Check sheet for the modelled part. Datum: model origin and axes. Units: mm. Face numbers are marked on the shaded views. A direction names the side the tool comes from. Give positions to 0.01 mm unless a question says otherwise; leave off trailing zeros. Loops run counter-clockwise (first coordinate to the right, second up) from the corner with the lowest first, then second, coordinate; pieces in that order, holes last. Notation, with made-up numbers: (-10, 68) - (37, 68) arc R24 cw to (37, 85) - close; hole circle Ø5 at (-39.75, -35.75). An arc over 180 degrees is marked (long way). Use CSV: the item, a comma, the result in double quotes.
from build123d import *

# Parameters (mm, degrees)
F0_R     = 2.3876
F1_DEPTH = 3.81
F2_R     = 2.3876
F3_DEPTH = 3.81
F4_SIZE  = 1.27


with BuildPart() as f1:
    # F0 (on Top) → F1 (new body)
    with BuildSketch(Plane.XY):
        with BuildLine():
            ThreePointArc((5.715, 9.7989101959), (0, 7.9772757461), (-5.715, 9.7989101959))
            Line((-5.715, 9.7989101959), (-5.715, 19.3437465092))
            Line((-5.715, 19.3437465092), (-7.6151215981, 19.3437465092))
            Line((-7.6151215981, 19.3437465092), (-9.3965170219, 13.432749836))
            Line((-9.3965170219, 13.432749836), (-9.3965170219, 6.983557897))
            Line((-9.3965170219, 6.983557897), (-4.1960714835, 1.5722833676))
            Line((-4.1960714835, 1.5722833676), (-4.1960714835, -12.9142534908))
            ThreePointArc((-4.1960714835, -12.9142534908), (-3.0057534422, -15.7879354495), (-0.1320714835, -16.9782534908))
            Line((-0.1320714835, -16.9782534908), (0, -16.9782534908))
            Line((0, -16.9782534908), (0.1320714835, -16.9782534908))
            ThreePointArc((0.1320714835, -16.9782534908), (3.0057534422, -15.7879354495), (4.1960714835, -12.9142534908))
            Line((4.1960714835, -12.9142534908), (4.1960714835, 1.5722833676))
            Line((4.1960714835, 1.5722833676), (9.3965170219, 6.983557897))
            Line((9.3965170219, 6.983557897), (9.3965170219, 13.432749836))
            Line((9.3965170219, 13.432749836), (7.6151215981, 19.3437465092))
            Line((7.6151215981, 19.3437465092), (5.715, 19.3437465092))
            Line((5.715, 19.3437465092), (5.715, 9.7989101959))
        make_face()
        with Locations((0, -11.8050774974)):
            Circle(F0_R, mode=Mode.SUBTRACT)
    extrude(amount=F1_DEPTH)

    # F2 (on face) → F3 (join)
    with BuildSketch(Plane.XY.offset(3.81)):
        with BuildLine():
            Line((-5.715, 9.7989101959), (-5.715, 19.3437465092))
            Line((-5.715, 19.3437465092), (-7.6151215981, 19.3437465092))
            Line((-7.6151215981, 19.3437465092), (-9.3965170219, 13.432749836))
            Line((-9.3965170219, 13.432749836), (-9.3965170219, 6.983557897))
            Line((-9.3965170219, 6.983557897), (-4.1960714835, 1.5722833676))
            Line((-4.1960714835, 1.5722833676), (-4.1960714835, -12.9142534908))
            ThreePointArc((-4.1960714835, -12.9142534908), (-3.0057534422, -15.7879354495), (-0.1320714835, -16.9782534908))
            Line((-0.1320714835, -16.9782534908), (0.1320714835, -16.9782534908))
            ThreePointArc((0.1320714835, -16.9782534908), (3.0057534422, -15.7879354495), (4.1960714835, -12.9142534908))
            Line((4.1960714835, -12.9142534908), (4.1960714835, 1.5722833676))
            Line((4.1960714835, 1.5722833676), (9.3965170219, 6.983557897))
            Line((9.3965170219, 6.983557897), (9.3965170219, 13.432749836))
            Line((9.3965170219, 13.432749836), (7.6151215981, 19.3437465092))
            Line((7.6151215981, 19.3437465092), (5.715, 19.3437465092))
            Line((5.715, 19.3437465092), (5.715, 9.7989101959))
            ThreePointArc((5.715, 9.7989101959), (0, 7.9772757461), (-5.715, 9.7989101959))
        make_face()
        with Locations((0, -11.8050774974)):
            Circle(F2_R, mode=Mode.SUBTRACT)
        with BuildLine():
            Line((-2.9692309909, 19.3437465092), (-5.715, 19.3437465092))
            Line((-5.715, 19.3437465092), (-5.715, 9.7989101959))
            ThreePointArc((-5.715, 9.7989101959), (0, 7.9772757461), (5.715, 9.7989101959))
            Line((5.715, 9.7989101959), (5.715, 19.3437465092))
            Line((5.715, 19.3437465092), (2.9692309909, 19.3437465092))
            Line((2.9692309909, 19.3437465092), (2.9692309909, 10.7184536755))
            Line((2.9692309909, 10.7184536755), (0, 10.7184536755))
            Line((0, 10.7184536755), (-2.9692309909, 10.7184536755))
            Line((-2.9692309909, 10.7184536755), (-2.9692309909, 19.3437465092))
        make_face()
    extrude(amount=F3_DEPTH)

    # F4
    f4_edges = [f1.edges().sort_by_distance(p)[0] for p in [
        (-8.505819, 16.388248, 7.62),
        (-9.396517, 10.208154, 7.62),
        (-6.796294, 4.277921, 7.62),
        (-4.196071, -5.670985, 7.62),
        (6.796294, 4.277921, 7.62),
        (9.396517, 10.208154, 7.62),
        (8.505819, 16.388248, 7.62),
    ]]
    chamfer(f4_edges, length=F4_SIZE)


solid = f1.part
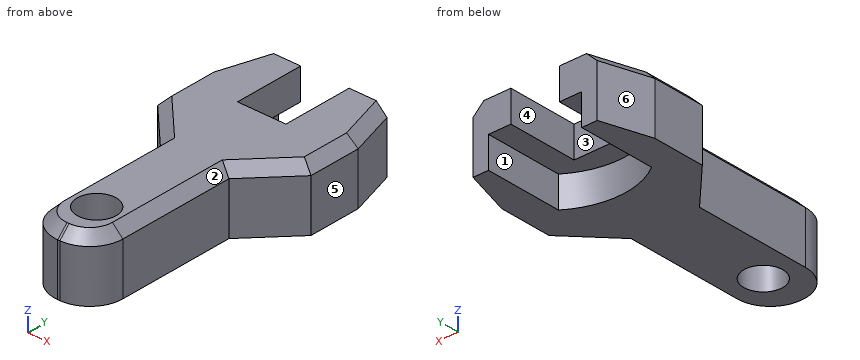
1. Scan lines: line 1 along Y through (x, z) = (0, 5.5); line 2 along X through (y, z) = (-12, 5); line 3 along Z through (x, y) = (-5.25, 12.5). Record each from-to range of solid material in increasing order.
Completed:
line 1,"y = -16.98 to -14.19, -9.42 to 10.72"
line 2,"x = -4.2 to -2.38, 2.38 to 4.2"
line 3,"z = 3.81 to 7.62"
2. Sectioned sample at A-A, the plane y = 15. Record the boundary of the cut face in (x, z) (3 decimals), and give its area (3 significant figures).
Completed:
outline,"(-8.924, 0) - (-5.715, 0) - (-5.715, 3.81) - (-2.969, 3.81) - (-2.969, 7.62) - (-7.598, 7.62) - (-8.924, 6.35) - close; (2.969, 3.81) - (5.715, 3.81) - (5.715, 0) - (8.924, 0) - (8.924, 6.35) - (7.598, 7.62) - (2.969, 7.62) - close"
area,"68.1 mm²"
3. Go/stop test with flat-tipped pins: pin 1 Ø5.5 at (x, y) = (0.5, 12) entering from -Z; pin 2 Ø1.1 at (y, z) = (16, 5) entering from +X; pin 3 Ø3 at (y, z) = (15, 1.5) entering from -X. Record where each tip stops, or that it passes through.
Completed:
pin 1,"stops at z = 3.81"
pin 2,"stops at x = 8.79"
pin 3,"stops at x = -9.38"
4. Sectioned sample at B-B, the plane y = -6. Record the boundary of the cut face in (x, z), and give its area (3 significant figures).
Completed:
outline,"(-4.2, 0) - (4.2, 0) - (4.2, 6.35) - (2.93, 7.62) - (-2.93, 7.62) - (-4.2, 6.35) - close"
area,"62.3 mm²"
5. Release check for a two-part mould opening along X. For the marked faces 4, 5 and 6 record: released by +X, released by -X, zero draft, split by the parting line, or undercut.
Completed:
face 4,"undercut"
face 5,"released by +X"
face 6,"released by -X"
6. Set-up check for the marked faces 1, 2 and 3: record each of +Z, -Z, +X, -X, +Y, -Y from which the full face is reachable in a straight line by a thin tool's end or side.
Completed:
face 1,"-Z, +Y"
face 2,"+Z, +X, -Y"
face 3,"+Z, -Z, +Y"
